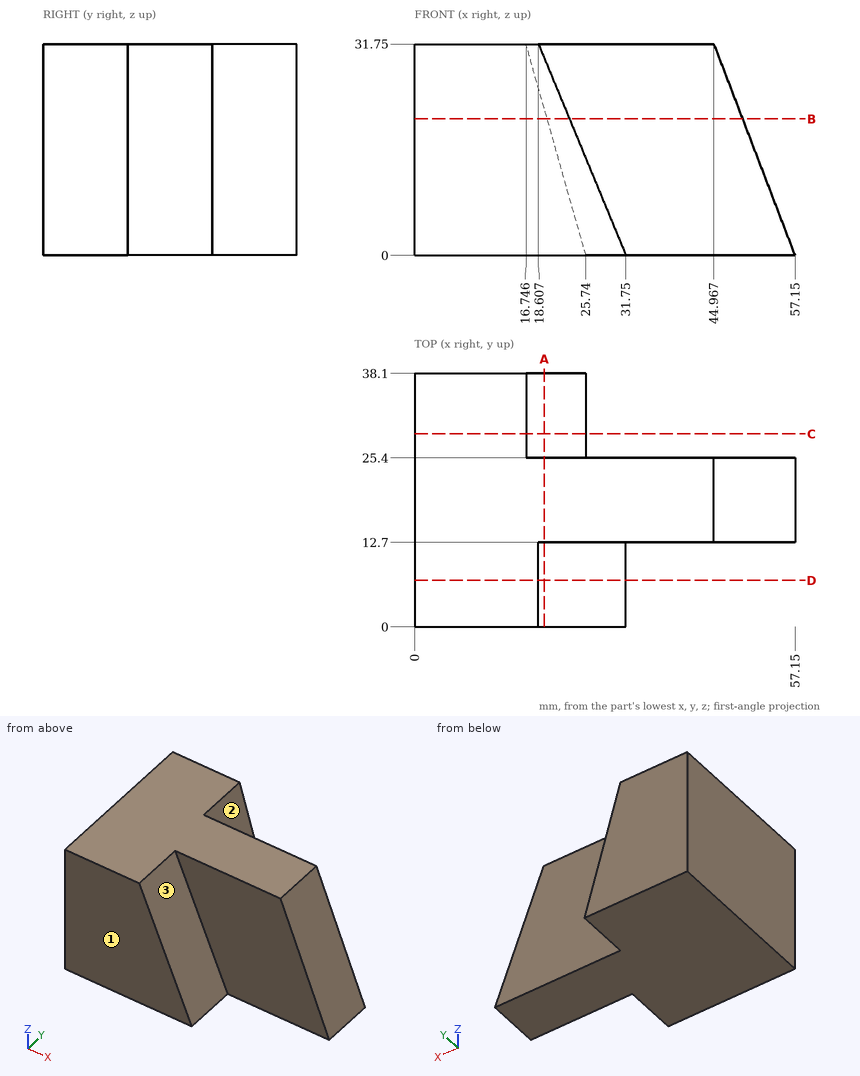
Part print with two shaded views. Sizes in mm from the minimum x, y, z corner. A direction names the side the tool comes from. Round coordinates to 2 decimals unless told otherwise and drop trailing zeros. Order: outer loops, then holes, each group sorted by start corner. A loop starts at its lowest first (then second) coordinate and runs counter-clockwise, first axis right, second up. Notation, with made-up numbers: M -28,14 L -22,14 A32 ccw -22,43 Z; hole C 24.5,75.25 d11. An arc over 180 degrees is marked long. Put each result on its own line as item: value. Start each with the question number.
1. Slice it at A-A on x = 19.5. List the corners of the cut face in (y, z), then the cut area to 3 significant figures.
2. Slice it at D-D on y = 7. List the corners of the cut face in (x, z).
3. Drill centre lines: probe 1 along Y at (x, z) = (26, 28.5); probe 2 along X at (y, z) = (5, 18.5); probe 3 along X at (y, z) = (27.5, 3.5). Where is each one in solid material? Low to high. Write a range as [from, to].
4. Drop flat-ended pins along their axis: pin 1 (2 mm diameter, centred on x = 26.5, z = 22, fed in from +Y); pin 2 (5 mm diameter, centred on y = 8, z = 15.5, fed in from +X); pin 3 (6 mm diameter, centred on x = 35, z = 23.5, fed in from -Y). Give the stop position or say it passes through.
5. Slice it at B-B on z = 20.5. List the corners of the cut face in (x, y).
6. Tool access for the marked faces 1, 2 and 3: list every direction of +Z, -Z, +X, -X, +Y, -Y with a clear straight run to the whole face (end or side of a thin tool).
7. Slice it at C-C on y = 29. List the corners of the cut face in (x, z).
Findings:
1. outline: M 0,0 L 38.1,0 L 38.1,22.03 L 25.4,22.03 L 25.4,31.75 L 12.7,31.75 L 12.7,29.59 L 0,29.59 Z
1. area: 1,060 mm2
2. outline: M 0,0 L 31.75,0 L 18.61,31.75 L 0,31.75 Z
3. probe 1: [12.7, 25.4]
3. probe 2: [0, 24.09]
3. probe 3: [0, 24.75]
4. pin 1: y = 25.4
4. pin 2: x = 26.37
4. pin 3: y = 12.7
5. outline: M 0,0 L 23.26,0 L 23.26,12.7 L 49.28,12.7 L 49.28,25.4 L 19.93,25.4 L 19.93,38.1 L 0,38.1 Z
6. face 1: +Z, -Z, +X, -X, -Y
6. face 2: +Z, +X, +Y
6. face 3: +Z, +X, -Y
7. outline: M 0,0 L 25.74,0 L 16.75,31.75 L 0,31.75 Z
